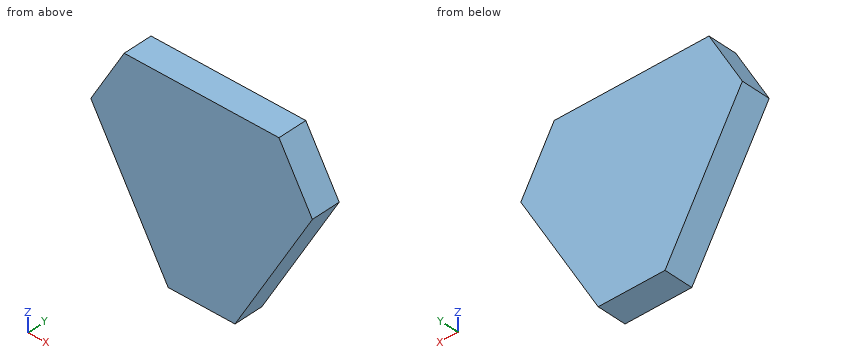
```python
from build123d import *

# Parameters (mm, degrees)
EXTRUDE_1_DEPTH     = 5
FILLET_1_R          = 20
EXTRUDE_2_DEPTH     = 10
SKETCH_3_W          = 458.835277925
SKETCH_3_H          = 325.644744519
CUT_EXTRUDE_1_DEPTH = 10


with BuildPart() as part:
    # 草圖1 → 填料-伸長1 (new body)
    with BuildSketch(Plane(origin=(0, 0, 0), x_dir=(1, 0, 0), z_dir=(0, 1, 0))):
        Polygon((-90.122176988, 0), (90.122176988, 0), (165.122176988, 129.903810568), (75, 286), (-75, 286), (-165.122176988, 129.903810568), align=None)
    extrude(amount=EXTRUDE_1_DEPTH)

    # 圓角1
    fillet_1_edges = [part.edges().sort_by_distance(p)[0] for p in [
        (-165.122176988, 2.5, -129.903810568),
        (-75, 2.5, -286),
        (75, 2.5, -286),
        (165.122176988, 2.5, -129.903810568),
        (90.122176988, 2.5, 0),
        (-90.122176988, 2.5, 0),
    ]]
    fillet(fillet_1_edges, radius=FILLET_1_R)

    # 草圖2 → 填料-伸長2 (add)
    with BuildSketch(Plane(origin=(0, 5, 0), x_dir=(1, 0, 0), z_dir=(0, 1, 0))):
        Polygon((-26.613647377, 110), (26.613647377, 110), (38.105117767, 129.903810568), (11.491470389, 176), (-11.491470389, 176), (-38.105117767, 129.903810568), align=None)
    extrude(amount=EXTRUDE_2_DEPTH)

    # 草圖3 → 除料-伸長1 (cut)
    with BuildSketch(Plane(origin=(0, 5, 0), x_dir=(1, 0, 0), z_dir=(0, 1, 0))):
        with Locations((11.913832117, 140.556137002)):
            Rectangle(SKETCH_3_W, SKETCH_3_H)
    extrude(amount=-CUT_EXTRUDE_1_DEPTH, mode=Mode.SUBTRACT)


solid = part.part
```
Read the model definition and answer for the solid it produces. Units are mm, in the model's axes. Give positions to 0.01 mm unless a question says otherwise; leave off trailing zeros. Loops run counter-clockwise (first coordinate to the right, second up) from the corner with the lowest first, then second, coordinate; pieces in that order, holes last.
Item 1: The part is cut by section C-C (x = 21). Write down the section's boundary in (y, z), and give its area (3 significant figures).
Item 2: The part is cut by section A-A (y = 6.75). Write down the section's boundary in (x, z).
Item 3: Find the intervals of material crossed by line 1 along X through (y, z) = (12, -147.5); line 2 along X through (y, z) = (12.75, -166.5); line 3 along Z through (x, y) = (33.5, 6.75), in increasing order.
Item 4: The part is cut by section B-B (z = -155). Write down the section's boundary in (x, y), and give its area (3 significant figures).
Item 5: Each of these flat-tipped pins is pushed along its axis until it touches: pin 1 Ø2 at (y, z) = (9.5, -133.5) entering from -X; pin 2 Ø1 at (y, z) = (11, -166.5) entering from -X (3 decimals). Where does it stop, or does it pass through?
Taken from the geometry:
1. outline: (5, -159.53) - (15, -159.53) - (15, -110) - (5, -110) - close
1. area: 495 mm2
2. outline: (-38.11, -129.9) - (-11.49, -176) - (11.49, -176) - (38.11, -129.9) - (26.61, -110) - (-26.61, -110) - close
3. line 1: x = -27.95 to 27.95
3. line 2: x = -16.98 to 16.98
3. line 3: z = -137.88 to -121.93
4. outline: (-23.62, 5) - (23.62, 5) - (23.62, 15) - (-23.62, 15) - close
4. area: 472 mm2
5. pin 1: stops at x = -36.61
5. pin 2: stops at x = -17.265
